Input: part model. Units: mm. Frame: model coordinates. Face numbers are marked on the shaded views. Coordinates: 2 decimals unless noted, no trailing zeros. Write each loop counter-clockwise with the first axis right and the second up, starting at its lowest first coordinate (ties: lowest second). Pieces come first, ordered by that corner, then holes.
1) Pin query (flat end, axial travel): pin 1 Ø6 at (x, z) = (-32.5, -18.5) entering from +Y; pin 2 Ø2 at (x, z) = (21, -21.5) entering from -Y; pin 3 Ø10 at (y, z) = (-51, -22.5) entering from +X; pin 4 Ø5 at (x, y) = (0, 15) entering from -Z. Return the tip coordinate at first contact, or that it passes through.
2) Line query: L1, parallel to Y at x = 48, z = -20.75; L2, parallel to Y at x = 50, z = -10.75; L3, parallel to Y at x = 2.5, z = -3.75. Output: solid intervals per line, ascending.
3) Section query D-D (x = 51). Output: boundary loops of the cut face in (y, z).
4) Section query A-A (z = -27.75). Output: boundary loops of the cut face in (x, y), then the cut area to 3 significant figures.
5) Section query C-C (y = 0). Output: boundary loops of the cut face in (x, z), then the cut area to 3 significant figures.
6) Draft query along Y for the marked faces 1, 2 and 3. Return one class per face: pulls with the +Y half, pulls with the -Y half, needs draft (parallel to the pull), parting line crosses it, or undercut.
7) Section query B-B (x = 0). Output: boundary loops of the cut face in (y, z).
Autodesk Inventor part; units mm, degrees
ref_plane "YZ Plane" through (0, 0, 0) normal (1, 0, 0) x (0, 1, 0)
ref_plane "XZ Plane" through (0, 0, 0) normal (0, 1, 0) x (-1, 0, 0)
ref_plane "XY Plane" through (0, 0, 0) normal (0, 0, 1) x (1, 0, 0)
ref_plane "Work Plane1" through (-40, 0, 12) normal (0, 1, 0) x (1, 0, 0)
sketch "Sketch2" plane through (-40, 0, 12) normal (0, 1, 0) x (1, 0, 0)
  line L0 (-30, 12) -> (110, 12)
  line L1 (40, 12) -> (40, 42)
  line L2 (40, 42) -> (110, 42)
  line L3 (110, 42) -> (110, 12)
  line L4 (110, 32) -> (104, 32)
  line L5 (104, 32) -> (104, 21)
  line L6 (104, 21) -> (110, 21)
  line L7 (110, 12) -> (40, 12)
  line L8 (40, 12) -> (40, 7)
  line L9 (40, 7) -> (110, 7)
  line L10 (110, 7) -> (110, 12)
  dimension "d3" = 30
  dimension "d4" = 10
  dimension "d5" = 11
  dimension "d6" = 6
  dimension "d17" = 5
revolve "Revolution1" add sketch "Sketch2" angle 360 about axis through (0, 0, 0) along (0, 0, -1) contours L1 L2 L3 L4 L5 L6 L0
sketch "Sketch3" plane through (0, 0, 0) normal (0, 0, 1) x (1, 0, 0)
  circle A0 centre (0, 0) radius 7.5
  dimension "d11" = 15
sketch "Sketch4" plane through (0, 0, 0) normal (0, 0, 1) x (1, 0, 0)
  circle A0 centre (50, 25) radius 2.05
  circle A1 centre (-50, -25) radius 2.05
  circle A2 centre (0, 15) radius 2.05
  circle A3 centre (50, -25) radius 2.05
  circle A4 centre (0, -15) radius 2.05
  circle A5 centre (-50, 25) radius 2.05
  line L0 (-40, 55) -> (40, 55)
  line L1 (40, 25) -> (40, 55)
  line L2 (40, 25) -> (-40, 25)
  line L3 (-40, 55) -> (-40, 25)
  line L4 (-40, -31) -> (40, -31)
  line L5 (40, -57.4456) -> (40, -31)
  arc A6 (40, -57.4456) -> (-40, -57.4456) centre (0, 0) ccw
  line L6 (-40, -31) -> (-40, -57.4456)
  circle A7 centre (-50, 25) radius 3
  circle A8 centre (-50, -25) radius 3
  circle A9 centre (0, -15) radius 3
  circle A10 centre (0, 15) radius 3
  circle A11 centre (50, 25) radius 3
  circle A12 centre (50, -25) radius 3
  dimension "d8" = 6
extrude "Extrusion2" cut sketch "Sketch4" against normal through all contours A0 | A1 | A2 | A3 | A4 | A5 | A7 | A8 | A9 | A10 | A11 | A12
extrude "Extrusion3" cut sketch "Sketch3" against normal blind 11
sketch "Sketch5" plane through (0, 0, -11) normal (0, 0, 1) x (1, 0, 0)
  circle A0 centre (0, 0) radius 2.75
  dimension "d14" = 5.5
extrude "Extrusion4" cut sketch "Sketch5" against normal through all
sketch "Sketch6" plane through (0, 0, 0) normal (0, 0, 1) x (1, 0, 0)
  point P0 (0, 0)
equation "\"BendRadius\" = Thickness"
equation "\"BendReliefWidth\" = Thickness"
equation "\"BendReliefDepth\" = 0.5 * Thickness"
equation "\"CornerReliefSize\" = 4 * Thickness"
equation "\"MinimumRemnant\" = 2 * Thickness"
equation "\"TransitionRadius\" = BendRadius"
equation "\"JacobiRadiusSize\" = BendRadius"
equation "\"GapSize\" = Thickness"
properties part number "base-top-plate_3DPrint"
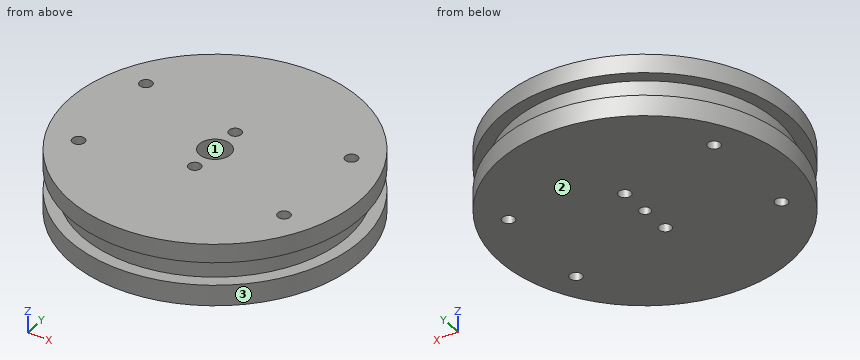
Answer:
1. pin 1: stops at y = 63.29
1. pin 2: stops at y = -67.08
1. pin 3: stops at x = 52.76
1. pin 4: passes through
2. L1: y = -50.95 to -27.24, -22.76 to 22.76, 27.24 to 50.95
2. L2: y = -39.95 to -28, -22 to 22, 28 to 39.95
2. L3: y = -69.96 to -16.66, -13.34 to -7.07, 7.07 to 13.34, 16.66 to 69.96
3. outline: (-47.95, -30) - (-27.83, -30) - (-27.83, 0) - (-47.95, 0) - (-47.95, -9) - (-38.67, -9) - (-38.67, -20) - (-47.95, -20) - close; (-22.17, -30) - (22.17, -30) - (22.17, 0) - (-22.17, 0) - close; (27.83, -30) - (47.95, -30) - (47.95, -20) - (38.67, -20) - (38.67, -9) - (47.95, -9) - (47.95, 0) - (27.83, 0) - close
4. outline: circle Ø140 at (0, 0); hole circle Ø6 at (-50, -25); hole circle Ø6 at (-50, 25); hole circle Ø6 at (0, -15); hole circle Ø6 at (0, 15); hole circle Ø5.5 at (0, 0); hole circle Ø6 at (50, -25); hole circle Ø6 at (50, 25)
4. area: 15,200 mm2
5. outline: (-70, -30) - (-2.75, -30) - (-2.75, -11) - (-7.5, -11) - (-7.5, 0) - (-70, 0) - (-70, -9) - (-64, -9) - (-64, -20) - (-70, -20) - close; (2.75, -30) - (70, -30) - (70, -20) - (64, -20) - (64, -9) - (70, -9) - (70, 0) - (7.5, 0) - (7.5, -11) - (2.75, -11) - close
5. area: 3,800 mm2
6. face 1: undercut
6. face 2: needs draft
6. face 3: parting line crosses it
7. outline: (-70, -30) - (-18, -30) - (-18, 0) - (-70, 0) - (-70, -9) - (-64, -9) - (-64, -20) - (-70, -20) - close; (-12, -30) - (-2.75, -30) - (-2.75, -11) - (-7.5, -11) - (-7.5, 0) - (-12, 0) - close; (2.75, -30) - (12, -30) - (12, 0) - (7.5, 0) - (7.5, -11) - (2.75, -11) - close; (18, -30) - (70, -30) - (70, -20) - (64, -20) - (64, -9) - (70, -9) - (70, 0) - (18, 0) - close
